from build123d import *

# Parameters (mm, degrees)
SKETCH1_W                       = 60.96
SKETCH1_H                       = 3.175
BOSS_EXTRUDE1_DEPTH             = 4.445
SKETCH3_R                       = 2.54
BOSS_EXTRUDE2_DEPTH             = 1.905
SKETCH4_W                       = 38.1
SKETCH4_H                       = 8.89
BOSS_EXTRUDE3_DEPTH             = 1.27
BOSS_EXTRUDE4_DEPTH             = 68.58
BOSS_EXTRUDE4_DEPTH_BACK        = 30.48
CUT_EXTRUDE1_DEPTH              = 2.905
CUT_EXTRUDE1_DEPTH_BACK         = 7.544579853
BOSS_EXTRUDE5_REACH             = 26.13
BOSS_EXTRUDE5_DIRECTION_2_REACH = 26.13
SKETCH9_W                       = 11.711761908
SKETCH9_H                       = 3.175
CUT_EXTRUDE2_DEPTH              = 3.328072262
CUT_EXTRUDE2_DEPTH_BACK         = 7.544579853
SKETCH10_R                      = 1.905
BOSS_EXTRUDE6_DEPTH             = 0.762
BOSS_EXTRUDE6_TAPER             = 45
SKETCH11_W                      = 58.42
SKETCH11_H                      = 5.08
CUT_EXTRUDE3_DEPTH              = 1.905
SKETCH12_R                      = 1.905
CUT_EXTRUDE5_DEPTH              = 2.54
SKETCH13_R                      = 1.905
SKETCH13_R_2                    = 0.9525
BOSS_EXTRUDE7_DEPTH             = 1.905


with BuildPart() as part:
    # Sketch1 → Boss-Extrude1 (new body, symmetric)
    with BuildSketch(Plane.XY):
        with Locations((0, -1.5875)):
            Rectangle(SKETCH1_W, SKETCH1_H)
    extrude(amount=BOSS_EXTRUDE1_DEPTH, both=True)

    # Sketch3 → Boss-Extrude2 (add)
    with BuildSketch(Plane(origin=(0, 0, 0), x_dir=(1, 0, 0), z_dir=(0, 1, 0))):
        with Locations((-25.4, 0)):
            Circle(SKETCH3_R)
        with Locations((-15.24, 0)):
            Circle(SKETCH3_R)
        with Locations((-5.08, 0)):
            Circle(SKETCH3_R)
        with Locations((5.08, 0)):
            Circle(SKETCH3_R)
        with Locations((15.24, 0)):
            Circle(SKETCH3_R)
        with Locations((25.4, 0)):
            Circle(SKETCH3_R)
    extrude(amount=BOSS_EXTRUDE2_DEPTH)

    # Sketch4 → Boss-Extrude3 (add)
    with BuildSketch(Plane(origin=(0, 0, 0), x_dir=(1, 0, 0), z_dir=(0, 1, 0))):
        with Locations((49.53, 0)):
            Rectangle(SKETCH4_W, SKETCH4_H)
    extrude(amount=-BOSS_EXTRUDE3_DEPTH)

    # Sketch5 → Boss-Extrude4 (add, two sides)
    with BuildSketch(Plane(origin=(0, 0, 0), x_dir=(0, 0, -1), z_dir=(1, 0, 0))) as boss_extrude4_sk:
        Polygon((4.445, 0), (24.13, -5.274579853), (24.13, -6.544579853), (4.445, -1.27), align=None)
        Polygon((-24.13, -6.544579853), (-24.13, -5.274579853), (-4.445, 0), (-4.445, -1.27), align=None)
    extrude(amount=BOSS_EXTRUDE4_DEPTH)
    extrude(boss_extrude4_sk.sketch, amount=-BOSS_EXTRUDE4_DEPTH_BACK)

    # Sketch7 → Cut-Extrude1 (cut, two sides)
    with BuildSketch(Plane(origin=(0, 0, 0), x_dir=(1, 0, 0), z_dir=(0, 1, 0))) as cut_extrude1_sk:
        Polygon((-30.48, 24.13), (-30.48, 4.445), (2.54, 24.13), align=None)
        Polygon((68.58, 24.13), (2.54, 24.13), (68.58, 4.445), align=None)
        Polygon((2.54, -24.13), (68.58, -4.445), (68.58, -24.13), align=None)
        Polygon((-30.48, -4.445), (-30.48, -24.13), (2.54, -24.13), align=None)
    extrude(amount=CUT_EXTRUDE1_DEPTH, mode=Mode.SUBTRACT)
    extrude(cut_extrude1_sk.sketch, amount=-CUT_EXTRUDE1_DEPTH_BACK, mode=Mode.SUBTRACT)

    # Boss-Extrude5: up to this face of the body (flat: up to its plane)
    boss_extrude5_end = Plane(part.part.faces().sort_by_distance((0, -2.2225, 4.445))[0])
    # Sketch8 → Boss-Extrude5 (add, up to the picked face)
    with BuildSketch(Plane.XY, mode=Mode.PRIVATE) as boss_extrude5_sk1:
        with BuildLine():
            Line((-30.48, -3.175), (-35.56, -3.175))
            ThreePointArc((-35.56, -3.175), (-35.822583927, -3.161390643), (-36.082353996, -3.120708411))
            Line((-36.082353996, -3.120708411), (-36.256100229, -3.598072262))
            Line((-36.256100229, -3.598072262), (-36.168460823, -3.10104449))
            ThreePointArc((-36.168460823, -3.10104449), (-36.455050568, -3.012074774), (-36.729147494, -2.889926637))
            Line((-36.729147494, -2.889926637), (-37.020524323, -3.306055875))
            Line((-37.020524323, -3.306055875), (-36.806879146, -2.847892314))
            ThreePointArc((-36.806879146, -2.847892314), (-37.096571594, -2.657510256), (-37.357643969, -2.429457066))
            Line((-37.357643969, -2.429457066), (-37.746641055, -2.755864377))
            Line((-37.746641055, -2.755864377), (-37.419184284, -2.365616595))
            ThreePointArc((-37.419184284, -2.365616595), (-37.915481622, -1.585424288), (-38.099614088, -0.679275117))
            Line((-38.099614088, -0.679275117), (-38.605680994, -0.635))
            Line((-38.605680994, -0.635), (-38.099614088, -0.590724883))
            ThreePointArc((-38.099614088, -0.590724883), (-37.915481622, 0.315424288), (-37.419184284, 1.095616595))
            Line((-37.419184284, 1.095616595), (-37.746641055, 1.485864377))
            Line((-37.746641055, 1.485864377), (-37.357643969, 1.159457066))
            ThreePointArc((-37.357643969, 1.159457066), (-37.096571594, 1.387510256), (-36.806879146, 1.577892314))
            Line((-36.806879146, 1.577892314), (-37.020524323, 2.036055875))
            Line((-37.020524323, 2.036055875), (-36.729147494, 1.619926637))
            ThreePointArc((-36.729147494, 1.619926637), (-36.455050568, 1.742074774), (-36.168460823, 1.83104449))
            Line((-36.168460823, 1.83104449), (-36.256100229, 2.328072262))
            Line((-36.256100229, 2.328072262), (-36.082353996, 1.850708411))
            ThreePointArc((-36.082353996, 1.850708411), (-35.822583927, 1.891390643), (-35.56, 1.905))
            Line((-35.56, 1.905), (-32.750290594, 1.905))
            Line((-32.750290594, 1.905), (-30.48, 0))
            Line((-30.48, 0), (-30.48, -3.175))
        make_face()
    boss_extrude5_tool1 = split(extrude(boss_extrude5_sk1.sketch, amount=BOSS_EXTRUDE5_REACH, mode=Mode.PRIVATE), bisect_by=boss_extrude5_end, keep=Keep.BOTH, mode=Mode.PRIVATE)
    add(boss_extrude5_tool1.solids().sort_by_distance((-34.232672, -0.756395, 0))[0])

    # Boss-Extrude5 direction 2: up to this face of the body (flat: up to its plane)
    boss_extrude5_direction_2_end = Plane(part.part.faces().sort_by_distance((0, -2.2225, -4.445))[0])
    # Sketch8 → Boss-Extrude5 direction 2 (add, up to the picked face)
    with BuildSketch(Plane.XY, mode=Mode.PRIVATE) as boss_extrude5_direction_2_sk1:
        with BuildLine():
            Line((-30.48, -3.175), (-35.56, -3.175))
            ThreePointArc((-35.56, -3.175), (-35.822583927, -3.161390643), (-36.082353996, -3.120708411))
            Line((-36.082353996, -3.120708411), (-36.256100229, -3.598072262))
            Line((-36.256100229, -3.598072262), (-36.168460823, -3.10104449))
            ThreePointArc((-36.168460823, -3.10104449), (-36.455050568, -3.012074774), (-36.729147494, -2.889926637))
            Line((-36.729147494, -2.889926637), (-37.020524323, -3.306055875))
            Line((-37.020524323, -3.306055875), (-36.806879146, -2.847892314))
            ThreePointArc((-36.806879146, -2.847892314), (-37.096571594, -2.657510256), (-37.357643969, -2.429457066))
            Line((-37.357643969, -2.429457066), (-37.746641055, -2.755864377))
            Line((-37.746641055, -2.755864377), (-37.419184284, -2.365616595))
            ThreePointArc((-37.419184284, -2.365616595), (-37.915481622, -1.585424288), (-38.099614088, -0.679275117))
            Line((-38.099614088, -0.679275117), (-38.605680994, -0.635))
            Line((-38.605680994, -0.635), (-38.099614088, -0.590724883))
            ThreePointArc((-38.099614088, -0.590724883), (-37.915481622, 0.315424288), (-37.419184284, 1.095616595))
            Line((-37.419184284, 1.095616595), (-37.746641055, 1.485864377))
            Line((-37.746641055, 1.485864377), (-37.357643969, 1.159457066))
            ThreePointArc((-37.357643969, 1.159457066), (-37.096571594, 1.387510256), (-36.806879146, 1.577892314))
            Line((-36.806879146, 1.577892314), (-37.020524323, 2.036055875))
            Line((-37.020524323, 2.036055875), (-36.729147494, 1.619926637))
            ThreePointArc((-36.729147494, 1.619926637), (-36.455050568, 1.742074774), (-36.168460823, 1.83104449))
            Line((-36.168460823, 1.83104449), (-36.256100229, 2.328072262))
            Line((-36.256100229, 2.328072262), (-36.082353996, 1.850708411))
            ThreePointArc((-36.082353996, 1.850708411), (-35.822583927, 1.891390643), (-35.56, 1.905))
            Line((-35.56, 1.905), (-32.750290594, 1.905))
            Line((-32.750290594, 1.905), (-30.48, 0))
            Line((-30.48, 0), (-30.48, -3.175))
        make_face()
    boss_extrude5_direction_2_tool1 = split(extrude(boss_extrude5_direction_2_sk1.sketch, amount=-BOSS_EXTRUDE5_DIRECTION_2_REACH, mode=Mode.PRIVATE), bisect_by=boss_extrude5_direction_2_end, keep=Keep.BOTH, mode=Mode.PRIVATE)
    add(boss_extrude5_direction_2_tool1.solids().sort_by_distance((-34.232672, -0.756395, 0))[0])

    # Sketch9 → Cut-Extrude2 (cut, two sides)
    with BuildSketch(Plane(origin=(0, 0, 0), x_dir=(1, 0, 0), z_dir=(0, 1, 0))) as cut_extrude2_sk:
        with Locations((-36.335880954, 0)):
            Rectangle(SKETCH9_W, SKETCH9_H)
    extrude(amount=CUT_EXTRUDE2_DEPTH, mode=Mode.SUBTRACT)
    extrude(cut_extrude2_sk.sketch, amount=-CUT_EXTRUDE2_DEPTH_BACK, mode=Mode.SUBTRACT)

    # Sketch10 → Boss-Extrude6 (add)
    with BuildSketch(Plane.XY.offset(-1.5875)):
        with Locations((-35.56, -0.635)):
            Circle(SKETCH10_R)
    boss_extrude6 = extrude(amount=BOSS_EXTRUDE6_DEPTH, taper=BOSS_EXTRUDE6_TAPER)

    # Mirror1: Boss-Extrude6 across plane
    add(boss_extrude6.mirror(Plane.XY))

    # Sketch11 → Cut-Extrude3 (cut)
    with BuildSketch(Plane.XZ.offset(3.175)):
        Rectangle(SKETCH11_W, SKETCH11_H)
    extrude(amount=-CUT_EXTRUDE3_DEPTH, mode=Mode.SUBTRACT)

    # Sketch12 → Cut-Extrude5 (cut)
    with BuildSketch(Plane.XZ.offset(1.27)):
        with Locations((-25.4, 0)):
            Circle(SKETCH12_R)
        with Locations((-15.24, 0)):
            Circle(SKETCH12_R)
        with Locations((-5.08, 0)):
            Circle(SKETCH12_R)
        with Locations((5.08, 0)):
            Circle(SKETCH12_R)
        with Locations((15.24, 0)):
            Circle(SKETCH12_R)
        with Locations((25.4, 0)):
            Circle(SKETCH12_R)
    extrude(amount=-CUT_EXTRUDE5_DEPTH, mode=Mode.SUBTRACT)

    # Sketch13 → Boss-Extrude7 (add)
    with BuildSketch(Plane.XZ.offset(1.27)):
        with Locations((-20.32, 0)):
            Circle(SKETCH13_R)
        with Locations((-20.32, 0)):
            Circle(SKETCH13_R_2, mode=Mode.SUBTRACT)
        with Locations((-10.16, 0)):
            Circle(SKETCH13_R)
        with Locations((-10.16, 0)):
            Circle(SKETCH13_R_2, mode=Mode.SUBTRACT)
        with Locations((10.16, 0)):
            Circle(SKETCH13_R)
        with Locations((10.16, 0)):
            Circle(SKETCH13_R_2, mode=Mode.SUBTRACT)
        with Locations((20.32, 0)):
            Circle(SKETCH13_R)
        with Locations((20.32, 0)):
            Circle(SKETCH13_R_2, mode=Mode.SUBTRACT)
        Circle(SKETCH13_R)
        Circle(SKETCH13_R_2, mode=Mode.SUBTRACT)
    extrude(amount=BOSS_EXTRUDE7_DEPTH)


solid = part.part
The listing builds one solid part. Answer for the finished solid, in the listing's coordinates (mm). A direction names the side the tool comes from. Coordinates: 2 decimals unless noted, no trailing zeros. Write each loop counter-clockwise with the first axis right and the second up, starting at its lowest first coordinate (ties: lowest second). Pieces come first, ordered by that corner, then holes. Notation, with made-up numbers: (-34.5, -11) - (14.5, -11) arc R32 cw to (14.5, 20) - close; hole circle Ø7 at (71, 50.25). An arc over 180 degrees is marked (long way). Return JSON: item names as keys, results as strings.
1. The part is cut by section A-A on x = -15.24. Determine the outline of the cut face in (y, z) (3 decimals).
Final values:
{"outline": "(-3.704, -13.53) - (-2.434, -13.53) - (0, -4.445) - (0, -2.54) - (1.905, -2.54) - (1.905, 2.54) - (0, 2.54) - (0, 4.445) - (-2.434, 13.53) - (-3.704, 13.53) - (-1.27, 4.445) - (-3.175, 4.445) - (-3.175, 2.54) - (-1.27, 2.54) - (-1.27, 1.905) - (1.27, 1.905) - (1.27, -1.905) - (-1.27, -1.905) - (-1.27, -2.54) - (-3.175, -2.54) - (-3.175, -4.445) - (-1.27, -4.445) - close"}
2. The part is cut by section D-D on x = 31.5. Determine the outline of the cut face in (y, z) (3 decimals).
Final values:
{"outline": "(-4.232, -15.498) - (-2.962, -15.498) - (0, -4.445) - (0, 4.445) - (-2.962, 15.498) - (-4.232, 15.498) - (-1.27, 4.445) - (-1.27, -4.445) - close"}
3. For a pull along X with two mould halves and no side action, classify faces 5 (the face through (23.497, -0.018, 0.084)), 6 (the face through (30.48, -2, 0)), 7 (the face through (-34, 1.905, 3)) as +X half, -X half, draft (parallel to the pull), parting line (faces both ways), or undercut.
Final values:
{"face 5": "undercut", "face 6": "+X half", "face 7": "draft"}
4. The part is cut by section B-B on x = 15.24. Determine the outline of the cut face in (y, z) (3 decimals), then the cut area to 3 significant figures.
Final values:
{"outline": "(-5.53, -20.344) - (-4.26, -20.344) - (0, -4.445) - (0, -2.54) - (1.905, -2.54) - (1.905, 2.54) - (0, 2.54) - (0, 4.445) - (-4.26, 20.344) - (-5.53, 20.344) - (-1.27, 4.445) - (-3.175, 4.445) - (-3.175, 2.54) - (-1.27, 2.54) - (-1.27, 1.905) - (1.27, 1.905) - (1.27, -1.905) - (-1.27, -1.905) - (-1.27, -2.54) - (-3.175, -2.54) - (-3.175, -4.445) - (-1.27, -4.445) - close", "area": "58.9 mm^2"}
5. Consider line 1 along Y through (x, z) = (25, -1) (3 decimals); line 2 along Y through (x, z) = (-28, 4) (3 decimals); line 3 along X through (y, z) = (-0.25, 3). Determine where each line is inside the solid, lowest interval first.
Final values:
{"line 1": "1.27 to 1.905", "line 2": "-3.175 to 0", "line 3": "-38.07 to 68.58"}
6. Which of the six approach directions +Z, -Z, +X, -X, +Y, -Y give full straight-line access (tool end or side, diameter ignored) to faces 1 (the face through (-12.817, 0.939, -0.763)), 2 (the face through (-33, -1, 1.588)), 3 (the face through (-0.21, -2.21, -0.93)), 4 (the face through (-31.631, 0.966, -2.996))?
Final values:
{"face 1": "+Y", "face 2": "none", "face 3": "-Y", "face 4": "+Z, -Z, +Y"}
7. Each of these flat-tipped pins is pushed along its axis until it touches: pin 1 Ø1.5 at (y, z) = (0, -11.5) entering from +X; pin 2 Ø4 at (x, z) = (-20.5, 0.5) entering from -Y (3 decimals); pin 3 Ø10 at (x, z) = (23, 2) entering from +Y (3 decimals); pin 4 Ø12 at (x, z) = (-12.5, 18) entering from +Y. Where does it stop, or does it pass through?
Final values:
{"pin 1": "through", "pin 2": "y = -3.175", "pin 3": "y = 1.905", "pin 4": "y = -2.02"}
8. The part is cut by section C-C on z = -6. Determine the outline of the cut face in (x, y).
Final values:
{"outline": "(-27.87, -1.69) - (63.36, -1.69) - (63.36, -0.42) - (-27.87, -0.42) - close"}
